Work out the finished part from the listing and answer in its coordinate system (mm). Face numbers are marked on the shaded views. A direction names the side the tool comes from. Coordinates: 2 decimals unless noted, no trailing zeros. Order: outer loops, then holes, each group sorted by start corner. A loop starts at its lowest first (then second) coordinate and runs counter-clockwise, first axis right, second up. Notation, with made-up numbers: M 88.5,6 L 113.5,6 A17 cw 113.5,17 Z; hole C -3,-40 d9. An arc over 180 degrees is marked long. Answer in a Markdown table with one row per item. Add a question column.
Item 1: A flat-ended cylindrical pin translates along its axis: pin 1 Ø1 at (x, y) = (-0.5, -0.5) entering from -Z. Find the tip coordinate at first contact, or state that the pin passes through.
Item 2: The part is cut by section B-B (x = 0). Write down the section's boundary in (y, z).
Item 3: Which of the six approach directions +Z, -Z, +X, -X, +Y, -Y give full straight-line access (tool end or side, diameter ignored) to the marked faces 4, 5 and 6?
Item 4: Consider line 1 (X direction, y = 0, z = 3.75); line 2 (X direction, y = 3, z = 2). Determine where each line is inside the solid, lowest interval first. Write a range as from..to.
Item 5: The mould has two halves that part along X. Classify the marked faces 1, 2 and 3: released by +X, released by -X, zero draft, split by the parting line, or undercut.
Item 6: The part is cut by section A-A (z = 7.75). Write down the section's boundary in (x, y).
from build123d import *

# Parameters (mm, degrees)
F0_W     = 15.8
F0_H     = 15.8
F1_DEPTH = 9.8
F2_R     = 2.4
F3_DEPTH = 1.8
F4_W     = 13.4
F4_H     = 13.4
F4_R     = 2.5
F4_R_2   = 1.75
F5_DEPTH = 8.9


with BuildPart() as f1:
    # F0 (on Top) → F1 (new body)
    with BuildSketch(Plane.XY):
        Rectangle(F0_W, F0_H)
    extrude(amount=F1_DEPTH)

    # F2 (on face) → F3 (join)
    with BuildSketch(Plane.XY.offset(9.8)):
        with Locations((-4.167743, 3.919162)):
            Circle(F2_R)
        with Locations((3.732257, 3.919162)):
            Circle(F2_R)
        with Locations((3.732257, -3.980838)):
            Circle(F2_R)
        with Locations((-4.167743, -3.980838)):
            Circle(F2_R)
    extrude(amount=F3_DEPTH)

    # F4 (on face) → F5 (cut)
    with BuildSketch(Plane(origin=(0, 0, 0), x_dir=(1, 0, 0), z_dir=(0, 0, -1))):
        Rectangle(F4_W, F4_H)
        Circle(F4_R, mode=Mode.SUBTRACT)
        Circle(F4_R_2)
    extrude(amount=-F5_DEPTH, mode=Mode.SUBTRACT)


solid = f1.part
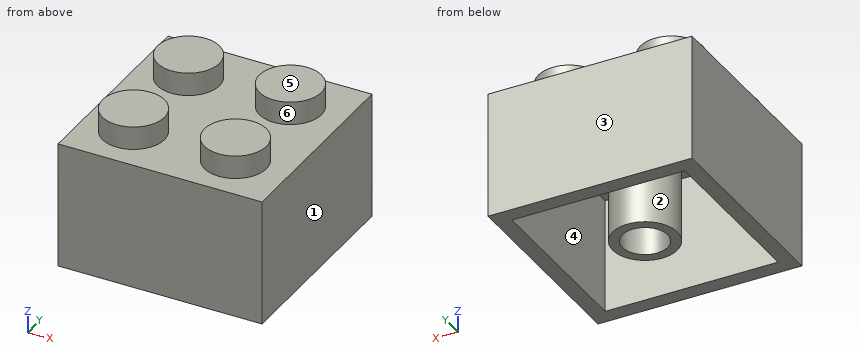
Reply:
| question | item | result |
|---|---|---|
| 1 | pin 1 | stops at z = 8.9 |
| 2 | outline | M -7.9,0 L -6.7,0 L -6.7,8.9 L -2.5,8.9 L -2.5,0 L -1.75,0 L -1.75,8.9 L 1.75,8.9 L 1.75,0 L 2.5,0 L 2.5,8.9 L 6.7,8.9 L 6.7,0 L 7.9,0 L 7.9,9.8 L -7.9,9.8 Z |
| 3 | face 4 | -Z |
| 3 | face 5 | +Z, +X, -X, +Y, -Y |
| 3 | face 6 | +Z |
| 4 | line 1 | x = -7.9..-6.7, -2.5..-1.75, 1.75..2.5, 6.7..7.9 |
| 4 | line 2 | x = -7.9..-6.7, 6.7..7.9 |
| 5 | face 1 | released by +X |
| 5 | face 2 | undercut |
| 5 | face 3 | zero draft |
| 6 | outline | M -7.9,-7.9 L 7.9,-7.9 L 7.9,7.9 L -7.9,7.9 Z; C 0,0 d5; hole M -6.7,-6.7 L 6.7,-6.7 L 6.7,6.7 L -6.7,6.7 Z; hole C 0,0 d3.5 |
